from build123d import *

# Parameters (mm, degrees)
F0_W     = 5
F0_H     = 8
F1_DEPTH = 25
F3_D     = 80.5
F4_R     = 5


with BuildPart() as f1:
    # F0 (on Top) → F1 (new body)
    with BuildSketch(Plane.XY):
        with Locations((-8.527812, 11.877605)):
            Rectangle(F0_W, F0_H)
    extrude(amount=F1_DEPTH)

    # F3 (through all)
    with Locations(Plane.YZ):
        with Locations((53.983625, 12.795336)):
            Hole(F3_D / 2)

    # F4
    f4_edges = [f1.edges().sort_by_distance(p)[0] for p in [
        (-8.527812, 7.877605, 0),
        (-8.527812, 7.877605, 25),
    ]]
    fillet(f4_edges, radius=F4_R)


solid = f1.part
The model under review builds one solid part; all positions refer to its coordinate system, in mm. Coordinates: 2 decimals unless noted, no trailing zeros. Loops run counter-clockwise (first coordinate to the right, second up) from the corner with the lowest first, then second, coordinate; pieces in that order, holes last. Notation, with made-up numbers: M -30,23 L 2,23 A15 ccw 2,27 Z; hole C 13,69 d2. An arc over 180 degrees is marked long. Put each result on its own line as item: value. Start each with the question number.
Q1. Add section C-C (z = 17.5). Write out the cut boundary in (x, y), and give its area (3 significant figures).
Q2. Add section D-D (y = 8.5). Write out the cut boundary in (x, z).
Q3. Wall thickness on line 1 (Y direction, x = -9.05, z = 12.5); line 2 (Y direction, x = -7.9, z = 20.25); line 3 (Z direction, x = -7.25, y = 11): over which ranges is each line inside the solid? List them lowest first.
Q4. Add section B-B (x = -7.05). Write out the cut boundary in (y, z).
Q5. Add section A-A (y = 15). Write out the cut boundary in (x, z).
Q6. Clearance check with a flat-ended pin moving along its axis: pin 1 (1.5 mm diameter, centred on x = -9.5, z = 18, fed in from +Y). State where the tip first meets the part, or that it passes through.
Answers:
1. outline: M -11.03,7.88 L -6.03,7.88 L -6.03,14.01 L -11.03,14.01 Z
1. area: 30.7 mm^2
2. outline: M -11.03,2.58 L -6.03,2.58 L -6.03,22.42 L -11.03,22.42 Z
3. line 1: y = 7.88 to 13.73
3. line 2: y = 7.88 to 14.43
3. line 3: z = 0.37 to 24.63
4. outline: M 7.88,5 A5 ccw 12.88,0 L 15.82,0 A40.25 cw 15.63,25 L 12.88,25 A5 ccw 7.88,20 Z
5. outline: M -11.03,0 L -6.03,0 L -6.03,2.78 L -11.03,2.78 Z; M -11.03,22.81 L -6.03,22.81 L -6.03,25 L -11.03,25 Z
6. pin 1: stops at y = 14.18
